from build123d import *

# Parameters (mm, degrees)
SKETCH2_R                  = 1.75
BOSS_EXTRUDE1_DEPTH        = 8
BOSS_EXTRUDE1_DEPTH_BACK   = 12
BOSS_EXTRUDE1_2_DEPTH      = 8
BOSS_EXTRUDE1_2_DEPTH_BACK = 12
BOSS_EXTRUDE1_3_DEPTH      = 8
BOSS_EXTRUDE1_3_DEPTH_BACK = 12
BOSS_EXTRUDE1_4_DEPTH      = 8
BOSS_EXTRUDE1_4_DEPTH_BACK = 12
SKETCH3_W                  = 77
SKETCH3_H                  = 60
SKETCH3_W_2                = 71
SKETCH3_H_2                = 54
BOSS_EXTRUDE2_DEPTH        = 8
SKETCH4_W                  = 77
SKETCH4_H                  = 60
BOSS_EXTRUDE3_DEPTH        = 3
CUT_EXTRUDE6_DEPTH         = 20
CUT_EXTRUDE8_DEPTH         = 13
CUT_EXTRUDE9_DEPTH         = 10
SKETCH17_R                 = 1
BOSS_EXTRUDE5_DEPTH        = 6
BOSS_EXTRUDE5_DEPTH_BACK   = 7
FILLET1_R                  = 1
BOSS_EXTRUDE6_DEPTH        = 11
FILLET3_R                  = 1
SKETCH20_R                 = 2.5
CUT_EXTRUDE10_DEPTH        = 10
SKETCH22_W                 = 34.401923789
SKETCH22_H                 = 2
CUT_EXTRUDE11_DEPTH        = 8


with BuildPart() as part:
    # Sketch2 → Boss-Extrude1 (new body, two sides)
    with BuildSketch(Plane.XY) as boss_extrude1_sk:
        with BuildLine():
            Line((-35.5, -27), (-25.5, -27))
            ThreePointArc((-25.5, -27), (-28.428932188, -19.928932188), (-35.5, -17))
            Line((-35.5, -17), (-35.5, -27))
        make_face()
        with Locations((-33, -23)):
            Circle(SKETCH2_R, mode=Mode.SUBTRACT)
    extrude(amount=BOSS_EXTRUDE1_DEPTH)
    extrude(boss_extrude1_sk.sketch, amount=-BOSS_EXTRUDE1_DEPTH_BACK)



with BuildPart() as body_2:
    # Sketch2 → Boss-Extrude1 2 (new body, two sides)
    with BuildSketch(Plane.XY) as boss_extrude1_2_sk:
        with BuildLine():
            Line((35.5, 27), (35.5, 17))
            ThreePointArc((35.5, 17), (28.428932188, 19.928932188), (25.5, 27))
            Line((25.5, 27), (35.5, 27))
        make_face()
        with Locations((33, 21)):
            Circle(SKETCH2_R, mode=Mode.SUBTRACT)
    extrude(amount=BOSS_EXTRUDE1_2_DEPTH)
    extrude(boss_extrude1_2_sk.sketch, amount=-BOSS_EXTRUDE1_2_DEPTH_BACK)


with BuildPart() as body_3:
    # Sketch2 → Boss-Extrude1 3 (new body, two sides)
    with BuildSketch(Plane.XY) as boss_extrude1_3_sk:
        with BuildLine():
            Line((-35.5, 27), (-25.5, 27))
            ThreePointArc((-25.5, 27), (-28.428932188, 19.928932188), (-35.5, 17))
            Line((-35.5, 17), (-35.5, 27))
        make_face()
        with Locations((-33, 21)):
            Circle(SKETCH2_R, mode=Mode.SUBTRACT)
    extrude(amount=BOSS_EXTRUDE1_3_DEPTH)
    extrude(boss_extrude1_3_sk.sketch, amount=-BOSS_EXTRUDE1_3_DEPTH_BACK)


with BuildPart() as body_4:
    # Sketch2 → Boss-Extrude1 4 (new body, two sides)
    with BuildSketch(Plane.XY) as boss_extrude1_4_sk:
        with BuildLine():
            Line((35.5, -17), (35.5, -27))
            Line((35.5, -27), (25.5, -27))
            ThreePointArc((25.5, -27), (28.428932188, -19.928932188), (35.5, -17))
        make_face()
        with Locations((33, -23)):
            Circle(SKETCH2_R, mode=Mode.SUBTRACT)
    extrude(amount=BOSS_EXTRUDE1_4_DEPTH)
    extrude(boss_extrude1_4_sk.sketch, amount=-BOSS_EXTRUDE1_4_DEPTH_BACK)


with BuildPart() as part_1:
    add(part.part)

    add(body_2.part)  # Boss-Extrude2 merges body 2

    add(body_3.part)  # Boss-Extrude2 merges body 3

    add(body_4.part)  # Boss-Extrude2 merges body 4
    # Sketch3 → Boss-Extrude2 (add)
    with BuildSketch(Plane.XY):
        Rectangle(SKETCH3_W, SKETCH3_H)
        Rectangle(SKETCH3_W_2, SKETCH3_H_2, mode=Mode.SUBTRACT)
    extrude(amount=BOSS_EXTRUDE2_DEPTH)

    # Sketch4 → Boss-Extrude3 (add)
    with BuildSketch(Plane.XY.offset(8)):
        Rectangle(SKETCH4_W, SKETCH4_H)
    extrude(amount=BOSS_EXTRUDE3_DEPTH)

    # Sketch12 → Cut-Extrude6 (cut)
    with BuildSketch(Plane(origin=(0, 0, -12), x_dir=(-1, 0, 0), z_dir=(0, 0, -1))):
        with BuildLine():
            Line((-35.5, -27), (-25.5, -27))
            ThreePointArc((-25.5, -27), (-28.428932188, -19.928932188), (-35.5, -17))
            Line((-35.5, -17), (-35.5, -27))
        make_face()
        with BuildLine():
            Line((35.5, -27), (35.5, -17))
            ThreePointArc((35.5, -17), (28.428932188, -19.928932188), (25.5, -27))
            Line((25.5, -27), (35.5, -27))
        make_face()
        with BuildLine():
            Line((35.5, 17), (35.5, 27))
            Line((35.5, 27), (25.5, 27))
            ThreePointArc((25.5, 27), (28.428932188, 19.928932188), (35.5, 17))
        make_face()
        with BuildLine():
            Line((-25.5, 27), (-35.5, 27))
            Line((-35.5, 27), (-35.5, 17))
            ThreePointArc((-35.5, 17), (-28.428932188, 19.928932188), (-25.5, 27))
        make_face()
    extrude(amount=-CUT_EXTRUDE6_DEPTH, mode=Mode.SUBTRACT)

    # Sketch14 → Cut-Extrude8 (cut)
    with BuildSketch(Plane(origin=(0, 30, 0), x_dir=(1, 0, 0), z_dir=(0, 1, 0))):
        with BuildLine():
            Line((22.5, -7.5), (15.5, -7.5))
            ThreePointArc((15.5, -7.5), (14.792893219, -7.207106781), (14.5, -6.5))
            Line((14.5, -6.5), (14.5, -3.5))
            ThreePointArc((14.5, -3.5), (14.792893219, -2.792893219), (15.5, -2.5))
            Line((15.5, -2.5), (22.5, -2.5))
            ThreePointArc((22.5, -2.5), (23.207106781, -2.792893219), (23.5, -3.5))
            Line((23.5, -3.5), (23.5, -6.5))
            ThreePointArc((23.5, -6.5), (23.207106781, -7.207106781), (22.5, -7.5))
        make_face()
    extrude(amount=-CUT_EXTRUDE8_DEPTH, mode=Mode.SUBTRACT)

    # Sketch15 → Cut-Extrude9 (cut)
    with BuildSketch(Plane.XY.offset(11)):
        with BuildLine():
            ThreePointArc((-0.027864045, -12), (-4.5, -10), (-8.972135955, -12))
            Line((-8.972135955, -12), (-0.027864045, -12))
        make_face()
        with BuildLine():
            Line((1.156854249, -14), (-10.156854249, -14))
            ThreePointArc((-10.156854249, -14), (-10.5, -16), (-10.156854249, -18))
            Line((-10.156854249, -18), (1.156854249, -18))
            ThreePointArc((1.156854249, -18), (1.413591358, -17.014611872), (1.5, -16))
            ThreePointArc((1.5, -16), (1.413591358, -14.985388128), (1.156854249, -14))
        make_face()
        with BuildLine():
            Line((-0.027864045, -20), (-8.972135955, -20))
            ThreePointArc((-8.972135955, -20), (-4.5, -22), (-0.027864045, -20))
        make_face()
    extrude(amount=-CUT_EXTRUDE9_DEPTH, mode=Mode.SUBTRACT)

    # Sketch17 → Boss-Extrude5 (add, two sides)
    with BuildSketch(Plane(origin=(0, 0, 0), x_dir=(-1, 0, 0), z_dir=(0, 0, -1))) as boss_extrude5_sk:
        with Locations((-37, 28.5)):
            Circle(SKETCH17_R)
        with Locations((37, 28.5)):
            Circle(SKETCH17_R)
        with Locations((37, -28.5)):
            Circle(SKETCH17_R)
        with Locations((-37, -28.472787798)):
            Circle(SKETCH17_R)
    extrude(amount=BOSS_EXTRUDE5_DEPTH)
    extrude(boss_extrude5_sk.sketch, amount=-BOSS_EXTRUDE5_DEPTH_BACK)

    # Fillet1
    fillet1_edges = [part_1.edges().sort_by_distance(p)[0] for p in [
        (-38.5, 30, 5.5),
        (38.5, 30, 5.5),
        (38.5, -30, 5.5),
        (-38.5, -30, 5.5),
    ]]
    fillet(fillet1_edges, radius=FILLET1_R)

    # Sketch19 → Boss-Extrude6 (add)
    with BuildSketch(Plane(origin=(0, 0, 0), x_dir=(-1, 0, 0), z_dir=(0, 0, -1))):
        with BuildLine():
            Line((38.5, 29), (38.5, 25.901923789))
            ThreePointArc((38.5, 25.901923789), (39.121320344, 30.621320344), (34.401923789, 30))
            Line((34.401923789, 30), (37.5, 30))
            ThreePointArc((37.5, 30), (38.207106781, 29.707106781), (38.5, 29))
        make_face()
        with BuildLine():
            Line((37.5, -30), (34.401923789, -30))
            ThreePointArc((34.401923789, -30), (39.121320344, -30.621320344), (38.5, -25.901923789))
            Line((38.5, -25.901923789), (38.5, -29))
            ThreePointArc((38.5, -29), (38.207106781, -29.707106781), (37.5, -30))
        make_face()
        with BuildLine():
            Line((-38.5, -29), (-38.5, -25.874711587))
            ThreePointArc((-38.5, -25.874711587), (-39.13243436, -30.582935589), (-34.417825937, -30))
            Line((-34.417825937, -30), (-37.5, -30))
            ThreePointArc((-37.5, -30), (-38.207106781, -29.707106781), (-38.5, -29))
        make_face()
        with BuildLine():
            Line((-37.5, 30), (-34.401923789, 30))
            ThreePointArc((-34.401923789, 30), (-39.121320344, 30.621320344), (-38.5, 25.901923789))
            Line((-38.5, 25.901923789), (-38.5, 29))
            ThreePointArc((-38.5, 29), (-38.207106781, 29.707106781), (-37.5, 30))
        make_face()
    extrude(amount=-BOSS_EXTRUDE6_DEPTH)

    # Fillet3
    fillet3_edges = [part_1.edges().sort_by_distance(p)[0] for p in [
        (-38.5, 0, 11),
        (-39.121320344, 30.621320344, 11),
        (0.007951074, -30, 11),
        (-39.121320344, -30.621320344, 11),
        (38.5, 0.013606101, 11),
        (39.13243436, -30.582935589, 11),
        (0, 30, 11),
        (39.121320344, 30.621320344, 11),
    ]]
    fillet(fillet3_edges, radius=FILLET3_R)

    # Sketch20 → Cut-Extrude10 (cut)
    with BuildSketch(Plane.XY.offset(11)):
        with Locations((-22.5, 14)):
            Circle(SKETCH20_R)
    extrude(amount=-CUT_EXTRUDE10_DEPTH, mode=Mode.SUBTRACT)

    # Sketch22 → Cut-Extrude11 (cut)
    with BuildSketch(Plane(origin=(0, 0, 0), x_dir=(-1, 0, 0), z_dir=(0, 0, -1))):
        with Locations((-17.200961895, 28)):
            Rectangle(SKETCH22_W, SKETCH22_H)
    extrude(amount=-CUT_EXTRUDE11_DEPTH, mode=Mode.SUBTRACT)


solid = part_1.part
Geometry check sheet. Reference: the model listing, model coordinates, mm. A direction names the side the tool comes from. Give positions to 0.01 mm unless a question says otherwise; leave off trailing zeros. Order: outer loops, then holes, each group sorted by start corner. A loop starts at its lowest first (then second) coordinate and runs counter-clockwise, first axis right, second up.
1) Cross-section at B-B (x = -22.5). Record the boundary of the cut face in (y, z), then the cut area to 3 significant figures.
Results are:
outline: (-30, 0) - (-27, 0) - (-27, 8) - (11.5, 8) - (11.5, 11) - (-29, 11) arc R1 ccw to (-30, 10) - close; (16.5, 8) - (27, 8) - (27, 0) - (30, 0) - (30, 10) arc R1 ccw to (29, 11) - (16.5, 11) - close
area: 213 mm2
2) Draft check along Y on faces 5 (the flat face through (0, 1, 8)), 6 (the flat face through (-37, 29, -6)). Enter one of: released by +Y, released by -Y, zero draft, split by the parting line, or undercut.
Results are:
face 5: undercut
face 6: zero draft
3) Cross-section at D-D (z = 5.5). Record the boundary of the cut face in (x, y), then the cut area to 3 significant figures.
Results are:
outline: (-38.5, -25.9) arc R3 ccw (long way) to (-34.4, -30) - (34.42, -30) arc R3 ccw (long way) to (38.5, -25.87) - (38.5, 25.9) arc R3 ccw (long way) to (34.4, 30) - (23.5, 30) - (23.5, 29) - (34.4, 29) - (34.4, 27) - (35.5, 27) - (35.5, -27) - (-35.5, -27) - (-35.5, 27) - (0, 27) - (0, 29) - (14.5, 29) - (14.5, 30) - (-34.4, 30) arc R3 ccw (long way) to (-38.5, 25.9) - close
area: 749 mm2
4) Tool access check on faces 1 (the flat face through (38.5, 0, 5)), 2 (the flat face through (-4, -20, 10)), 3 (the cylindrical face through (36.46, -27.63, -2.96)), 4 (the flat face through (37, 29, -6)). Record the directions out of +Z, -Z, +X, -X, +Y, -Y that give a thin tool (end or side, any length) a straight path to the whole face; none if there is none.
Results are:
face 1: +Z, -Z, +X
face 2: +Z, -Z
face 3: -Z
face 4: -Z, +X, -X, +Y, -Y
5) Cross-section at C-C (x = -5). Record the boundary of the cut face in (y, z).
Results are:
outline: (-30, 0) - (-27, 0) - (-27, 8) - (-21.98, 8) - (-21.98, 11) - (-29, 11) arc R1 ccw to (-30, 10) - close; (-20, 8) - (-18, 8) - (-18, 11) - (-20, 11) - close; (-14, 8) - (-12, 8) - (-12, 11) - (-14, 11) - close; (-10.02, 8) - (27, 8) - (27, 0) - (30, 0) - (30, 10) arc R1 ccw to (29, 11) - (-10.02, 11) - close
6) Cross-section at A-A (y = 14). Record the boundary of the cut face in (x, z), then the cut area to 3 significant figures.
Results are:
outline: (-38.5, 0) - (-35.5, 0) - (-35.5, 8) - (-25, 8) - (-25, 11) - (-37.5, 11) arc R1 ccw to (-38.5, 10) - close; (-20, 8) - (35.5, 8) - (35.5, 0) - (38.5, 0) - (38.5, 10) arc R1 ccw to (37.5, 11) - (-20, 11) - close
area: 264 mm2
7) Gauge pin test, flat ends, axial feed: pin 1 (3.5 mm diameter, centred on x = -3.5, z = 9.5, fed in from -Y); pin 2 (10 mm diameter, centred on x = 27, z = -3, fed in from +Y); pin 3 (9 mm diameter, centred on y = -1.5, z = 4, fed in from -X). Record the tip position at first contact, or that the pin passes through.
Results are:
pin 1: stops at y = -30
pin 2: stops at y = 30
pin 3: stops at x = -38.5
8) Material ranges on probe 1 along Y at (x, z) = (30, 2.5); probe 2 along X at (y, z) = (-4, 3); probe 3 along Y at (x, z) = (-22.5, 9.3), recorded low to high.
Results are:
probe 1: y = -30 to -27, 29 to 30
probe 2: x = -38.5 to -35.5, 35.5 to 38.5
probe 3: y = -30 to 11.5, 16.5 to 30
